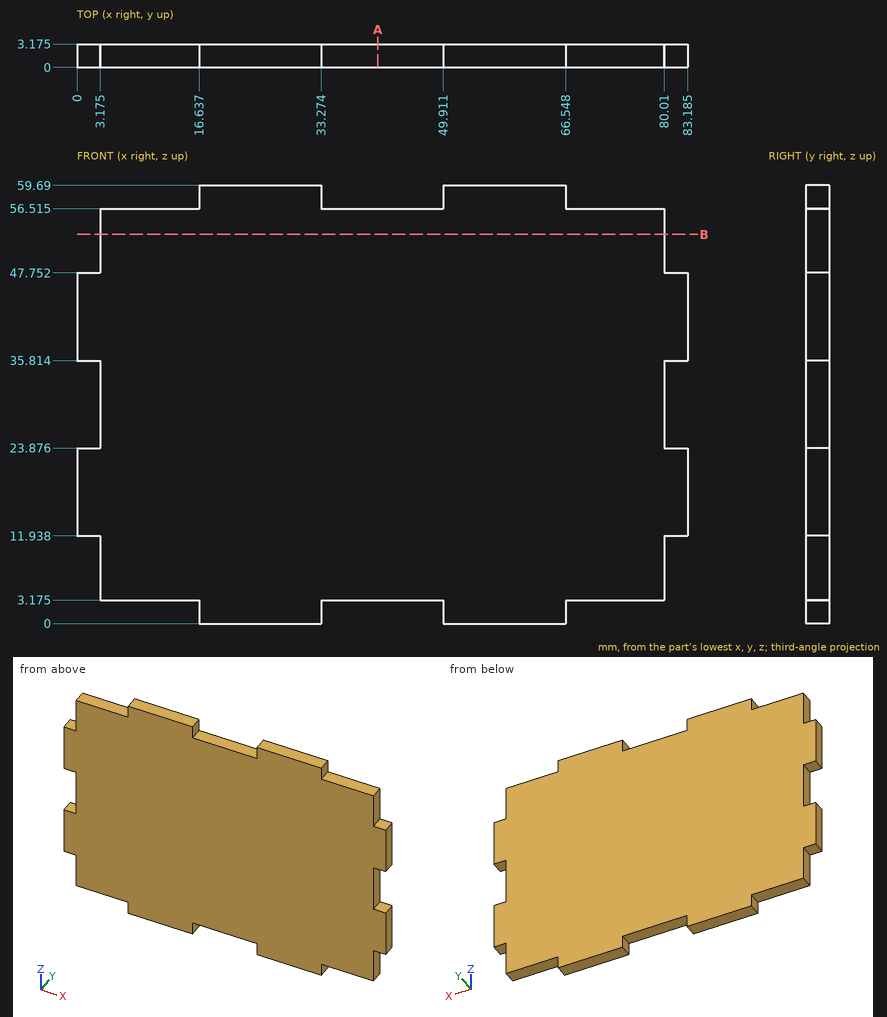
Geometry: see drawing. Coordinates: mm, zero at the bounding-box minimum. Give positions to 0.01 mm unless a question says otherwise; leave off trailing zeros. Loops run counter-clockwise (first coordinate to the right, second up) from the corner with the lowest first, then second, coordinate; pieces in that order, holes last. Notation, with made-up numbers: (7, -7.5) - (56, -7.5) arc R37 cw to (56, 28.5) - close; hole circle Ø1 at (83, 6). An arc over 180 degrees is marked (long way). One line per question, with ' | ' between items. Start each with the question number.
(1) Contact query for flat-ended pins moving along their axis: pin 1 (1.6 mm diameter, centred on y = 2, z = 58, fed in from +X); pin 2 (1.5 mm diameter, centred on x = 37.5, y = 2.5, fed in from +Z) (3 decimals); pin 3 (1 mm diameter, centred on x = 13, y = 1, fed in from -Z) (3 decimals). Output: stop coordinate, or through.
(2) Section query A-A on x = 41. Return loops of the section in (y, z) (3 decimals).
(3) Ray query, line 1 (Z direction, x = 38.5, y = 1.4) (3 decimals); line 2 (X direction, y = 2.85, z = 26) (3 decimals). Return the intervals inside material, ascending. Write a range as from..to.
(4) Section query B-B on z = 53. Return loops of the section in (x, y) (3 decimals).
The answers:
1) pin 1: x = 66.55 | pin 2: z = 56.515 | pin 3: z = 3.175
2) outline: (0, 3.175) - (3.175, 3.175) - (3.175, 56.515) - (0, 56.515) - close
3) line 1: 3.175..56.515 | line 2: 3.175..80.01
4) outline: (3.175, 0) - (80.01, 0) - (80.01, 3.175) - (3.175, 3.175) - close
